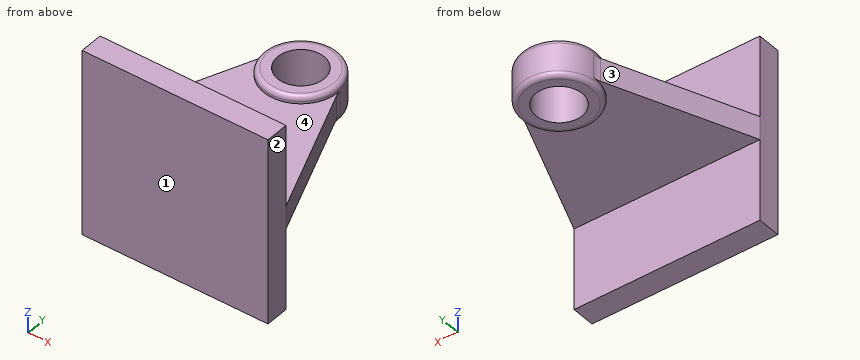
```python
from build123d import *

# Parameters (mm, degrees)
SKETCH1_W           = 50.8
SKETCH1_H           = 50.8
BOSS_EXTRUDE1_DEPTH = 6.35
SKETCH2_R           = 10.16
SKETCH2_R_2         = 6.35
BOSS_EXTRUDE2_DEPTH = 5.08
BOSS_EXTRUDE3_DEPTH = 3.175
FILLET3_R           = 6.35


with BuildPart() as part:
    # Sketch1 → Boss-Extrude1 (new body)
    with BuildSketch(Plane(origin=(0, 0, 0), x_dir=(1, 0, 0), z_dir=(0, 1, 0))):
        Rectangle(SKETCH1_W, SKETCH1_H)
    extrude(amount=BOSS_EXTRUDE1_DEPTH)



with BuildPart() as body_2:
    # Sketch2 → Boss-Extrude2 (new, symmetric)
    with BuildSketch(Plane.XY):
        with Locations((0, 44.45)):
            Circle(SKETCH2_R)
        with Locations((0, 44.45)):
            Circle(SKETCH2_R_2, mode=Mode.SUBTRACT)
    extrude(amount=BOSS_EXTRUDE2_DEPTH, both=True)


with BuildPart() as part_1:
    add(part.part)

    add(body_2.part)  # Boss-Extrude3 merges body 2
    # Sketch4 → Boss-Extrude3 (add, symmetric)
    with BuildSketch(Plane.XY):
        with BuildLine():
            Line((-10.16, 44.45), (-25.4, 6.35))
            Line((-25.4, 6.35), (25.4, 6.35))
            Line((25.4, 6.35), (10.16, 44.45))
            ThreePointArc((10.16, 44.45), (0, 34.29), (-10.16, 44.45))
        make_face()
    extrude(amount=BOSS_EXTRUDE3_DEPTH, both=True)

    # Fillet2: read off the stored shape, not the designer's step
    # Fillet2 outline → Fillet2 (revolve, cut)
    with BuildSketch(Plane.XZ.offset(-44.45)):
        with BuildLine():
            ThreePointArc((10.16, -3.81), (9.788025612, -4.708025612), (8.89, -5.08))
            Line((8.89, -5.08), (10.16, -5.08))
            Line((10.16, -5.08), (10.16, -3.81))
        make_face()
        with BuildLine():
            ThreePointArc((8.89, 5.08), (9.788025612, 4.708025612), (10.16, 3.81))
            Line((10.16, 3.81), (10.16, 5.08))
            Line((10.16, 5.08), (8.89, 5.08))
        make_face()
    revolve(axis=Axis((0, 44.45, 0), (0, 0, 1)), mode=Mode.SUBTRACT)

    # Fillet3
    # the kernel refuses this fillet: 6.35 mm, written as the material it adds along each edge
    with BuildSketch(Plane(origin=(10.16, 44.45, 3.175), x_dir=(-0.041343675933645734, 0.9991449847045691, 0), z_dir=(0, 0, -1))) as fillet3_piece_1:
        with BuildLine():
            CenterArc((1.102635837, 6.344570653), FILLET3_R, 250.56808401, 17.062422493)
            Line((-1.009923388, 0.356282624), (0, 0))
            ThreePointArc((0, 0), (0.420051747, 0.008686955), (0.840103495, 0))
        make_face()
    extrude(amount=6.35)
    with BuildSketch(Plane(origin=(-10.16, 44.45, 3.175), x_dir=(0.04134367593364538, 0.9991449847045691, 0), z_dir=(0, 0, -1))) as fillet3_piece_2:
        with BuildLine():
            CenterArc((1.102635837, -6.344570653), FILLET3_R, 92.369493497, 17.062422493)
            Line((-1.009923388, -0.356282624), (0, 0))
            ThreePointArc((0, 0), (0.420051747, -0.008686955), (0.840103495, 0))
        make_face()
    extrude(amount=6.35)


solid = part_1.part
```
Build history of the part. All positions in model axes, mm. Face numbers are marked on the shaded views. Give positions to 0.01 mm unless a question says otherwise; leave off trailing zeros. Loops run counter-clockwise (first coordinate to the right, second up) from the corner with the lowest first, then second, coordinate; pieces in that order, holes last.
Item 1: Slice it at A-A, the plane x = 0. List the corners of the cut face in (y, z) (3 decimals).
Answers follow:
outline: (0, -25.4) - (6.35, -25.4) - (6.35, -3.175) - (34.29, -3.175) - (34.29, -3.81) arc R1.27 ccw to (35.56, -5.08) - (38.1, -5.08) - (38.1, 5.08) - (35.56, 5.08) arc R1.27 ccw to (34.29, 3.81) - (34.29, 3.175) - (6.35, 3.175) - (6.35, 25.4) - (0, 25.4) - close; (50.8, -5.08) - (53.34, -5.08) arc R1.27 ccw to (54.61, -3.81) - (54.61, 3.81) arc R1.27 ccw to (53.34, 5.08) - (50.8, 5.08) - close
Item 2: Drill centre lines: line 1 (Y direction, x = 0, z = -3); line 2 (Y direction, x = 18.5, z = 4); line 3 (Z direction, x = -19.5, y = 11) (3 decimals). Where is each one in solid material? Low to high.
Answers follow:
line 1: y = 0 to 38.1, 50.8 to 54.61
line 2: y = 0 to 6.35
line 3: z = -3.175 to 3.175
Item 3: Slice it at B-B, the plane z = 2. List the corners of the cut face in (x, y), and give its area (3 significant figures).
Answers follow:
outline: (-25.4, 0) - (25.4, 0) - (25.4, 6.35) - (10.56, 43.46) arc R6.35 cw to (10.13, 45.29) arc R10.16 ccw to (-10.13, 45.29) arc R6.35 cw to (-10.56, 43.46) - (-25.4, 6.35) - close; hole circle Ø12.7 at (0, 44.45)
area: 1,710 mm2
Item 4: Flat gauge pins, fed straight in: pin 1 (8 mm diameter, centred on x = -13.5, y = 48, fed in from +Z); pin 2 (9 mm diameter, centred on x = 1.5, y = 42.5, fed in from +Z); pin 3 (8 mm diameter, centred on x = 16, z = -11, fed in from -Y); pin 4 (19.5 mm diameter, centred on x = 3.5, y = 45.5, fed in from -Z). Where does each tip first touch, or does it go through?
Answers follow:
pin 1: stops at z = 4.5
pin 2: stops at z = 5.08
pin 3: stops at y = 0
pin 4: stops at z = -5.08
Item 5: Slice it at D-D, the plane y = 44.45. List the corners of the cut face in (x, z) (3 decimals).
Answers follow:
outline: (-10.252, -3.175) - (-10.16, -3.175) - (-10.16, -3.81) arc R1.27 ccw to (-8.89, -5.08) - (-6.35, -5.08) - (-6.35, 5.08) - (-8.89, 5.08) arc R1.27 ccw to (-10.16, 3.81) - (-10.16, 3.175) - (-10.252, 3.175) - close; (6.35, -5.08) - (8.89, -5.08) arc R1.27 ccw to (10.16, -3.81) - (10.16, -3.175) - (10.252, -3.175) - (10.252, 3.175) - (10.16, 3.175) - (10.16, 3.81) arc R1.27 ccw to (8.89, 5.08) - (6.35, 5.08) - close
Item 6: Slice it at C-C, the plane x = 18. List the corners of the cut face in (y, z) (3 decimals), and give its area (3 significant figures).
Answers follow:
outline: (0, -25.4) - (6.35, -25.4) - (6.35, -3.175) - (24.85, -3.175) - (24.85, 3.175) - (6.35, 3.175) - (6.35, 25.4) - (0, 25.4) - close
area: 440 mm2
Item 7: Pull direction Y, two halves, no side cores. Call the marked faces 1, 2, 3 and 4: released by +Y, released by -Y, zero draft, split by the parting line, or undercut.
Answers follow:
face 1: released by -Y
face 2: zero draft
face 3: released by +Y
face 4: undercut
